from build123d import *

# Parameters (mm, degrees)
SKETCH_2_R      = 4
EXTRUDE_1_DEPTH = 11.36
EXTRUDE_2_DEPTH = 102
SKETCH_4_R      = 3.42
EXTRUDE_3_DEPTH = 22


with BuildPart() as part:
    # 草图1 → 旋转1 (revolve)
    with BuildSketch(Plane.XY, mode=Mode.PRIVATE) as revolve_1_sk:
        Polygon((0, 0), (7.5, 0), (42.09, 53.35), (42.09, 76.73), (49.525, 76.73), (49.525, 95.5), (62.215, 95.5), (62.215, 104.91), (54.51, 104.91), (54.51, 107.98), (43.65, 107.98), (43.65, 142.98), (39.635, 142.98), (39.635, 246.28), (42.62, 246.28), (42.62, 233.91), (76.8, 233.91), (76.8, 244.9), (63.67, 244.9), (63.67, 275.1), (49.47, 275.1), (49.47, 356.23), (66.395, 356.23), (66.395, 381.8), (49.47, 381.8), (49.47, 404.27), (66.395, 404.27), (66.395, 422.79), (39.72, 422.79), (39.72, 432.61), (76.34, 432.61), (76.34, 448.79), (55.36, 448.79), (55.36, 478.82), (76.34, 478.82), (76.34, 490.29), (61.69, 490.29), (61.69, 546.17), (58.9, 546.17), (58.9, 628.71), (63.765, 628.71), (63.765, 678.34), (80.93, 678.34), (80.93, 690.98), (58.9, 690.98), (58.9, 633.2), (34.64, 633.2), (34.64, 422.88), (0, 422.88), align=None)
    revolve(revolve_1_sk.sketch.rotate(Axis((0, 0, 0), (0, 1, 0)), 90), axis=Axis((0, 0, 0), (0, 1, 0)))

    # 草图2 → 凸台-拉伸1 (add)
    with BuildSketch(Plane(origin=(0, 422.88, 0), x_dir=(1, 0, 0), z_dir=(0, 1, 0))):
        with Locations(Location((0, 0, 0), (0, 0, 90))):
            Circle(SKETCH_2_R)
    extrude(amount=EXTRUDE_1_DEPTH)

    # 草图3 → 凸台-拉伸2 (add)
    with BuildSketch(Plane(origin=(0, 434.24, 0), x_dir=(1, 0, 0), z_dir=(0, 1, 0))):
        Polygon((7.349668927, 0), (3.674834463, 6.365), (-3.674834463, 6.365), (-7.349668927, 0), (-3.674834463, -6.365), (3.674834463, -6.365), align=None)
    extrude(amount=EXTRUDE_2_DEPTH)

    # 草图4 → 凸台-拉伸3 (add)
    with BuildSketch(Plane(origin=(0, 536.24, 0), x_dir=(1, 0, 0), z_dir=(0, 1, 0))):
        with Locations(Location((0, 0, 0), (0, 0, 270))):
            Circle(SKETCH_4_R)
    extrude(amount=EXTRUDE_3_DEPTH)


solid = part.part
Verification items for the finished model (mm, model axes). A direction names the side the tool comes from. Give positions to 0.01 mm unless a question says otherwise; leave off trailing zeros. Loops run counter-clockwise (first coordinate to the right, second up) from the corner with the lowest first, then second, coordinate; pieces in that order, holes last.
1. Cross-section at B-B on y = 199. Record the cut outline in (x, z) (3 decimals).
Derived:
outline: circle Ø79.27 at (0, 0)
2. Material ranges on probe 1 along X at (y, z) = (539, 0); probe 2 along Y at (x, z) = (58.5, -41); probe 3 along X at (y, z) = (472, 0), recorded low to high.
Derived:
probe 1: x = -61.69 to -34.64, -3.42 to 3.42, 34.64 to 61.69
probe 2: y = 233.91 to 244.9, 432.61 to 448.79, 478.82 to 490.29, 678.34 to 690.98
probe 3: x = -55.36 to -34.64, -7.35 to 7.35, 34.64 to 55.36
3. Release check for a two-part mould opening along Y. For faces 6 (the conical face through (16.938, 15.193, 3.761)), 7 (the cylindrical face through (-12.643, 65.204, -40.146)), 8 (the flat face through (3, 434.24, -3)) record: +Y half, -Y half, draft (parallel to the pull), parting line (faces both ways), or undercut.
Derived:
face 6: -Y half
face 7: draft
face 8: undercut
4. Cross-section at C-C on y = 88.5. Record the cut outline in (x, z) (3 decimals), and give its area (3 significant figures).
Derived:
outline: circle Ø99.05 at (0, 0)
area: 7,710 mm2
5. Go/stop test with flat-tipped pins: P1, Ø1.5, axis at x = -50, z = -63.5, coming from the -Y side; P2, Ø12, axis at x = 14.5, y = 147, coming from the +Z side; P3, Ø12, axis at x = -58, y = 250, coming from the -Z side. Record where each tip stops, or that it passes through.
Derived:
P1: stops at y = 678.34
P2: stops at z = 42.48
P3: stops at z = -53.77
6. Tool access check on faces 1 (the flat face through (60, 690.98, -6)), 2 (the flat face through (0, 0, 0)), 3 (the flat face through (-24, 678.34, 60)), 4 (the flat face through (27, 95.5, -42)), 5 (the flat face through (3, 536.24, -2)). Record the directions out of +Z, -Z, +X, -X, +Y, -Y that give a thin tool (end or side, any length) a straight path to the whole face; none if there is none.
Derived:
face 1: +Z, -Z, +X, -X, +Y
face 2: +Z, -Z, +X, -X, -Y
face 3: none
face 4: -Y
face 5: +Y
7. Cross-section at A-A on y = 465. Record the cut outline in (x, z) (3 decimals).
Derived:
outline: circle Ø110.72 at (0, 0); (-7.35, 0) - (-3.675, -6.365) - (3.675, -6.365) - (7.35, 0) - (3.675, 6.365) - (-3.675, 6.365) - close; hole circle Ø69.28 at (0, 0)
